Part model, mm, in its own coordinate system. A direction names the side the tool comes from. Round coordinates to 2 decimals unless told otherwise and drop trailing zeros. Write each loop counter-clockwise with the first axis right and the second up, starting at its lowest first coordinate (ties: lowest second). Pieces come first, ordered by that corner, then holes.
```python
from build123d import *

# Parameters (mm, degrees)
SKETCH1_W           = 14
SKETCH1_H           = 22
SKETCH1_W_2         = 10
SKETCH1_H_2         = 18
EXTRUDE_THIN1_DEPTH = 2
SKETCH2_W           = 2
SKETCH2_H           = 22
BOSS_EXTRUDE1_DEPTH = 4.5
SKETCH3_W           = 22
SKETCH3_H           = 8
SKETCH3_W_2         = 18
SKETCH3_H_2         = 4
EXTRUDE_THIN2_DEPTH = 2
SKETCH4_W           = 2
SKETCH4_H           = 10.076871622
CUT_EXTRUDE1_DEPTH  = 26.690465157
SKETCH5_W           = 1.1
SKETCH5_H           = 4.2
SKETCH5_H_2         = 2
CUT_EXTRUDE2_DEPTH  = 1.1
BOSS_EXTRUDE2_DEPTH = 8
SKETCH7_W           = 2.5
SKETCH7_H           = 1.1
SKETCH7_W_2         = 0.9
BOSS_EXTRUDE3_DEPTH = 8
CUT_EXTRUDE3_DEPTH  = 1.1
BOSS_EXTRUDE4_REACH = 25.065
SKETCH9_W           = 2
SKETCH9_H           = 4
BOSS_EXTRUDE5_DEPTH = 2
SKETCH11_W          = 0.9
SKETCH11_H          = 4.2
BOSS_EXTRUDE6_DEPTH = 1.1
EXTRUDE_THIN4_DEPTH = 2
LPATTERN1_COUNT     = 2
LPATTERN1_PITCH     = 18
SKETCH14_W          = 2.2
SKETCH14_H          = 4.2
CUT_EXTRUDE4_DEPTH  = 2
FILLET1_R           = 1


with BuildPart() as part:
    # Sketch1 → Extrude-Thin1 (new body)
    with BuildSketch(Plane(origin=(0, 0, 0), x_dir=(1, 0, 0), z_dir=(0, 1, 0))):
        with Locations((5, 9)):
            Rectangle(SKETCH1_W, SKETCH1_H)
        with Locations((5, 9)):
            Rectangle(SKETCH1_W_2, SKETCH1_H_2, mode=Mode.SUBTRACT)
    extrude(amount=EXTRUDE_THIN1_DEPTH)

    # Sketch2 → Boss-Extrude1 (add)
    with BuildSketch(Plane(origin=(0, 2, 0), x_dir=(1, 0, 0), z_dir=(0, 1, 0))):
        with Locations((11, 9)):
            Rectangle(SKETCH2_W, SKETCH2_H)
    extrude(amount=BOSS_EXTRUDE1_DEPTH)

    # Sketch3 → Extrude-Thin2 (add)
    with BuildSketch(Plane.ZY.offset(2)):
        with Locations((-9, 4)):
            Rectangle(SKETCH3_W, SKETCH3_H)
        with Locations((-9, 4)):
            Rectangle(SKETCH3_W_2, SKETCH3_H_2, mode=Mode.SUBTRACT)
    extrude(amount=-EXTRUDE_THIN2_DEPTH)

    # Sketch4 → Cut-Extrude1 (cut, through all)
    with BuildSketch(Plane(origin=(12, 0, 0), x_dir=(0, 0, -1), z_dir=(1, 0, 0))):
        with Locations((19, 5.038435811)):
            Rectangle(SKETCH4_W, SKETCH4_H)
    extrude(amount=-CUT_EXTRUDE1_DEPTH, mode=Mode.SUBTRACT)

    # Sketch5 → Cut-Extrude2 (cut)
    with BuildSketch(Plane(origin=(0, 0, -18), x_dir=(-1, 0, 0), z_dir=(0, 0, -1))):
        with Locations((-11.45, 3)):
            Rectangle(SKETCH5_W, SKETCH5_H)
        with Locations((1.45, 7)):
            Rectangle(SKETCH5_W, SKETCH5_H_2)
        with Locations((1.45, 1)):
            Rectangle(SKETCH5_W, SKETCH5_H_2)
    extrude(amount=-CUT_EXTRUDE2_DEPTH, mode=Mode.SUBTRACT)

    # Sketch6 → Boss-Extrude2 (add)
    with BuildSketch(Plane.ZY.offset(2)):
        Polygon((-16.9, 2), (-16.9, 0), (2, 0), (2, 8), (-16.9, 8), (-16.9, 6), (0, 6), (0, 2), align=None)
    extrude(amount=BOSS_EXTRUDE2_DEPTH)

    # Sketch7 → Boss-Extrude3 (add, through all)
    with BuildSketch(Plane(origin=(0, 8, 0), x_dir=(1, 0, 0), z_dir=(0, 1, 0))):
        with Locations((-2.15, 17.45)):
            Rectangle(SKETCH7_W, SKETCH7_H)
        with Locations((-7.85, 17.45)):
            Rectangle(SKETCH7_W, SKETCH7_H)
        with Locations((-9.55, 17.45)):
            Rectangle(SKETCH7_W_2, SKETCH7_H)
    extrude(amount=-BOSS_EXTRUDE3_DEPTH)

    # Sketch8 → Cut-Extrude3 (cut)
    with BuildSketch(Plane(origin=(0, 0, -18), x_dir=(-1, 0, 0), z_dir=(0, 0, -1))):
        Polygon((6.6, 6), (0.9, 6), (0.9, 2), (6.6, 4.505494505), align=None)
        Polygon((6.6, 4.505494505), (0.9, 2), (6.6, 2), align=None)
        Polygon((10, 2), (10, 6), (6.6, 4.505494505), (6.6, 2), align=None)
        Polygon((10, 6), (6.6, 6), (6.6, 4.505494505), align=None)
    extrude(amount=-CUT_EXTRUDE3_DEPTH, mode=Mode.SUBTRACT)

    # Sketch9 → Boss-Extrude4 (add, up to next)
    with BuildSketch(Plane(origin=(0, 0, 0), x_dir=(0, 0, -1), z_dir=(1, 0, 0)), mode=Mode.PRIVATE) as boss_extrude4_sk1:
        with Locations((-1, 4)):
            Rectangle(SKETCH9_W, SKETCH9_H)
    boss_extrude4_tool1 = extrude(boss_extrude4_sk1.sketch, amount=BOSS_EXTRUDE4_REACH, mode=Mode.PRIVATE) - part.part
    add(boss_extrude4_tool1.solids().sort_by_distance((0, 4, 1))[0])

    # Sketch10 → Boss-Extrude5 (add)
    with BuildSketch(Plane(origin=(12, 0, 0), x_dir=(0, 0, -1), z_dir=(1, 0, 0))):
        Polygon((-2, 6.5), (-2, 0), (18, 0), (18, 0.9), (16.9, 0.9), (16.9, 5.1), (18, 5.1), (18, 6.5), align=None)
    extrude(amount=BOSS_EXTRUDE5_DEPTH)

    # Sketch11 → Boss-Extrude6 (add)
    with BuildSketch(Plane(origin=(0, 0, -16.9), x_dir=(-1, 0, 0), z_dir=(0, 0, -1))):
        with Locations((-13.55, 3)):
            Rectangle(SKETCH11_W, SKETCH11_H)
    extrude(amount=BOSS_EXTRUDE6_DEPTH)

    # Sketch13 → Extrude-Thin4 (add)
    with BuildSketch(Plane.XY.offset(2)):
        Polygon((-10, 0), (-10, -13.856406461), (14, 0), (13, 1.732050808), (-8, -10.392304845), (-8, 0), align=None)
    extrude_thin4 = extrude(amount=-EXTRUDE_THIN4_DEPTH)

    # LPattern1: Extrude-Thin4 ×2
    with Locations(*[(0, 0, -i * LPATTERN1_PITCH) for i in range(1, LPATTERN1_COUNT)]):
        add(extrude_thin4)

    # Sketch14 → Cut-Extrude4 (cut)
    with BuildSketch(Plane(origin=(0, 0, -16.9), x_dir=(-1, 0, 0), z_dir=(0, 0, -1))):
        with Locations((-12, 3)):
            Rectangle(SKETCH14_W, SKETCH14_H)
    extrude(amount=CUT_EXTRUDE4_DEPTH, mode=Mode.SUBTRACT)

    # Fillet1
    # the kernel refuses this fillet: 1 mm, written as the material it adds along each edge
    with BuildSketch(Plane(origin=(10, 0, 0), x_dir=(-0.866025403784438, -0.500000000000001, 0), z_dir=(0, 0, 1))) as fillet1_piece_1:
        with BuildLine():
            CenterArc((FILLET1_R * 3.73205080757, -FILLET1_R), FILLET1_R, 90, 150)
            Line((FILLET1_R * 3.23205080757, -FILLET1_R * 1.86602540378), (0, 0))
            Line((0, 0), (FILLET1_R * 3.73205080757, 0))
        make_face()
    extrude(amount=2)
    with BuildSketch(Plane(origin=(-8, -10.392304845, 2), x_dir=(0.8660254037844376, 0.5000000000000017, 0), z_dir=(0, 0, -1))) as fillet1_piece_2:
        with BuildLine():
            CenterArc((FILLET1_R * 1.73205080757, -FILLET1_R), FILLET1_R, 90, 120)
            Line((FILLET1_R * 0.866025403784, -FILLET1_R * 1.5), (0, 0))
            Line((0, 0), (FILLET1_R * 1.73205080757, 0))
        make_face()
    extrude(amount=2)
    with BuildSketch(Plane(origin=(-8, 0, 2), x_dir=(0, -1, 0), z_dir=(0, 0, -1)), Plane(origin=(-8, 0, -16), x_dir=(0, -1, 0), z_dir=(0, 0, -1))) as fillet1_piece_3:
        with BuildLine():
            CenterArc((FILLET1_R, -FILLET1_R), FILLET1_R, 90, 90)
            Line((0, -FILLET1_R), (0, 0))
            Line((0, 0), (FILLET1_R, 0))
        make_face()
    extrude(amount=2)
    with BuildSketch(Plane(origin=(10, 0, -16), x_dir=(0, 1, 0), z_dir=(0, 0, -1))) as fillet1_piece_4:
        with BuildLine():
            CenterArc((FILLET1_R * 0.57735026919, -FILLET1_R), FILLET1_R, 90, 60)
            Line((-FILLET1_R * 0.288675134595, -FILLET1_R * 0.5), (0, 0))
            Line((0, 0), (FILLET1_R * 0.57735026919, 0))
        make_face()
    extrude(amount=2)
    with BuildSketch(Plane(origin=(-8, -10.392304845, -16), x_dir=(0, 1, 0), z_dir=(0, 0, -1))) as fillet1_piece_5:
        with BuildLine():
            CenterArc((FILLET1_R * 1.73205080757, FILLET1_R), FILLET1_R, 150, 120)
            Line((FILLET1_R * 0.866025403784, FILLET1_R * 1.5), (0, 0))
            Line((0, 0), (FILLET1_R * 1.73205080757, 0))
        make_face()
    extrude(amount=2)
    # the kernel refuses this fillet: 1 mm, written as the material it takes off along each edge
    with BuildSketch(Plane(origin=(0, 0, -20.5), x_dir=(-1, 0, 0), z_dir=(0, 0, 1)), Plane(origin=(-10, 2, 0), x_dir=(0, -1, 0), z_dir=(0, 0, -1))) as fillet1_2_piece_1:
        with BuildLine():
            CenterArc((FILLET1_R, -FILLET1_R), FILLET1_R, 90, 90)
            Line((0, -FILLET1_R), (0, 0))
            Line((0, 0), (FILLET1_R, 0))
        make_face()
    extrude(amount=20.5, mode=Mode.SUBTRACT)
    with BuildSketch(Plane(origin=(0, 2, -20.5), x_dir=(-1, 0, 0), z_dir=(0, 0, 1)), Plane(origin=(-10, 6, -20.5), x_dir=(1, 0, 0), z_dir=(0, 0, 1)), Plane(origin=(0, 6, 0), x_dir=(-1, 0, 0), z_dir=(0, 0, -1))) as fillet1_2_piece_2:
        with BuildLine():
            CenterArc((FILLET1_R, FILLET1_R), FILLET1_R, 180, 90)
            Line((0, FILLET1_R), (0, 0))
            Line((0, 0), (FILLET1_R, 0))
        make_face()
    extrude(amount=20.5, mode=Mode.SUBTRACT)
    with BuildSketch(Plane(origin=(-10, 8, 4.5), x_dir=(1, 0, 0), z_dir=(0, 0, -1)), Plane(origin=(14, 6.5, -20.5), x_dir=(-1, 0, 0), z_dir=(0, 0, 1))) as fillet1_2_piece_3:
        with BuildLine():
            CenterArc((FILLET1_R, FILLET1_R), FILLET1_R, 180, 90)
            Line((0, FILLET1_R), (0, 0))
            Line((0, 0), (FILLET1_R, 0))
        make_face()
    extrude(amount=25, mode=Mode.SUBTRACT)
    with BuildSketch(Plane(origin=(-10, -13.856406461, 6.330127019), x_dir=(0.866025403784438, 0.5000000000000009, 0), z_dir=(0, 0, -1))) as fillet1_2_piece_4:
        with BuildLine():
            CenterArc((FILLET1_R * 1.73205080757, -FILLET1_R), FILLET1_R, 90, 120)
            Line((FILLET1_R * 0.866025403784, -FILLET1_R * 1.5), (0, 0))
            Line((0, 0), (FILLET1_R * 1.73205080757, 0))
        make_face()
    extrude(amount=10.660254038, mode=Mode.SUBTRACT)
    with BuildSketch(Plane(origin=(0, 8, 4.5), x_dir=(-1, 0, 0), z_dir=(0, 0, -1))) as fillet1_2_piece_5:
        with BuildLine():
            CenterArc((FILLET1_R, -FILLET1_R), FILLET1_R, 90, 90)
            Line((0, -FILLET1_R), (0, 0))
            Line((0, 0), (FILLET1_R, 0))
        make_face()
    extrude(amount=25, mode=Mode.SUBTRACT)
    with BuildSketch(Plane(origin=(10, 6.5, -20.5), x_dir=(1, 0, 0), z_dir=(0, 0, 1))) as fillet1_2_piece_6_section:
        with BuildLine():
            CenterArc((FILLET1_R, -FILLET1_R), FILLET1_R, 90, 90)
            Line((0, -FILLET1_R), (0, 0))
            Line((0, 0), (FILLET1_R, 0))
        make_face()
    fillet1_2_piece_6 = extrude(amount=25, mode=Mode.PRIVATE)
    fillet1_2_piece_6 = split(fillet1_2_piece_6, bisect_by=Plane(origin=(10.244024849, 6, -9), z_dir=(0, 1, 0)), keep=Keep.TOP, mode=Mode.PRIVATE)
    add(fillet1_2_piece_6, mode=Mode.SUBTRACT)
    with BuildSketch(Plane(origin=(10, 6.5, -20.5), x_dir=(1, 0, 0), z_dir=(0, 0, 1))) as fillet1_2_piece_7_section:
        with BuildLine():
            CenterArc((FILLET1_R, -FILLET1_R), FILLET1_R, 90, 90)
            Line((0, -FILLET1_R), (0, 0))
            Line((0, 0), (FILLET1_R, 0))
        make_face()
    fillet1_2_piece_7 = extrude(amount=25, mode=Mode.PRIVATE)
    fillet1_2_piece_7 = split(fillet1_2_piece_7, bisect_by=Plane(origin=(10.039684593, 5.876736387, 0), z_dir=(0, 0, -1)), keep=Keep.TOP, mode=Mode.PRIVATE)
    add(fillet1_2_piece_7, mode=Mode.SUBTRACT)
    with BuildSketch(Plane(origin=(-10, 0, 0), x_dir=(1, 0, 0), z_dir=(0, 0, -1))) as fillet1_2_piece_8:
        with BuildLine():
            CenterArc((FILLET1_R, -FILLET1_R), FILLET1_R, 90, 90)
            Line((0, -FILLET1_R), (0, 0))
            Line((0, 0), (FILLET1_R, 0))
        make_face()
    extrude(amount=16, mode=Mode.SUBTRACT)
    with BuildSketch(Plane(origin=(-10, -13.856406461, -11.669872981), x_dir=(0, 1, 0), z_dir=(0, 0, -1))) as fillet1_2_piece_9:
        with BuildLine():
            CenterArc((FILLET1_R * 1.73205080757, FILLET1_R), FILLET1_R, 150, 120)
            Line((FILLET1_R * 0.866025403784, FILLET1_R * 1.5), (0, 0))
            Line((0, 0), (FILLET1_R * 1.73205080757, 0))
        make_face()
    extrude(amount=10.660254038, mode=Mode.SUBTRACT)


solid = part.part
```
Q1. Cut at B-B on y = -10. Write the cut outline in (x, z).
Values follow:
outline: (-10, -18) - (-3.32, -18) - (-3.32, -16) - (-10, -16) - close; (-10, 0) - (-3.32, 0) - (-3.32, 2) - (-10, 2) - close
Q2. Cut at A-A on z = -10. Write the cut outline in (x, y), plus the area to 3 significant figures.
Values follow:
outline: (-9, 0) - (-1, 0) arc R1 ccw to (-1, 2) - (-9, 2) arc R1 ccw to start; (-9, 6) - (-1, 6) arc R1 ccw to (-1, 8) - (-9, 8) arc R1 ccw to start; (10, 0) - (14, 0) - (14, 5.5) arc R1 ccw to (13, 6.5) - (11, 6.5) arc R1 ccw to (10, 5.5) - close
area: 63.9 mm2
Q3. Wall check: L1, parallel to Y at x = 11.25, z = -10.75; L2, parallel to Z at x = 2.75, y = 3; L3, parallel to X at y = 3.25, z = -11. Give the ranges that are in metal, low to high.
Values follow:
L1: y = 0 to 6.5
L2: z = 0 to 2
L3: x = 10 to 14
Q4. Drop flat-ended pins along their axis: pin 1 (6.5 mm diameter, centred on x = -3, z = -10.5, fed in from -Y); pin 2 (8 mm diameter, centred on x = 5.5, y = 5, fed in from -Z); pin 3 (1.2 mm diameter, centred on x = 12.5, z = -17.5, fed in from -Y). Give the stop position or say it passes through.
Values follow:
pin 1: stops at y = 0
pin 2: stops at z = 0
pin 3: stops at y = -1.21
Q5. Cut at C-C on x = 0.75. Write the cut outline in (y, z), plus the area to 3 significant figures.
Values follow:
outline: (-7.65, -18) - (-5.34, -18) - (-5.34, -16) - (-7.65, -16) - close; (-7.65, 0) - (-5.34, 0) - (-5.34, 2) - (-7.65, 2) - close; (0, 0) - (6, 0) - (6, 2) - (0, 2) - close
area: 21.2 mm2
Q6. Cut at D-D on y = 4. Write the cut outline in (x, z), plus the area to 3 significant figures.
Values follow:
outline: (-10, 0) - (10, 0) - (10, -18) - (10.9, -18) - (10.9, -16.9) - (13.1, -16.9) - (13.1, -18) - (14, -18) - (14, 2) - (-10, 2) - close
area: 118 mm2
Q7. Which spindle directions (+Z, -Z, +X, -X, +Y, -Y) get a long thin tool onto all of the face, cutting with end or side? Do faces 5 (the flat face through (-5, 2, -9)), 6 (the flat face through (1.612, -4.843, -16.986)), 7 (the flat face through (-5, 8, -8)), 8 (the flat face through (-8, -5, 1)), 9 (the flat face through (-3.4, 7, -17.4)). Say none if no direction does.
Values follow:
face 5: -Z, -X
face 6: -Z
face 7: +Z, -Z, +X, -X, +Y
face 8: +Z, -Z
face 9: -Z, +Y
Q8. Mould opens along X. For faces 1 (the flat face through (5, 6, 1)), 2 (the flat face through (-10, -2, 1)), 3 (the flat face through (-8, 7, -18)), 4 (the flat face through (2.592, -6.586, 1.014)) say: +X half, -X half, draft (parallel to the pull), parting line (faces both ways), or undercut.
Values follow:
face 1: undercut
face 2: -X half
face 3: draft
face 4: +X half
